from build123d import *

# Parameters (mm, degrees)
F1_DEPTH = 25.4
F3_DEPTH = 25.4
F4_W     = 29.7458320856
F4_H     = 10.7239410281
F4_W_2   = 77.620446682
F4_W_3   = 25.7802940905
F4_H_2   = 64.6573156118
F4_W_4   = 82.3989063501
F4_H_3   = 15.7408937812
F4_W_5   = 43.0548340082
F4_H_4   = 22.1842341125
F4_W_6   = 2.0285844803
F4_H_5   = 2.3600235581
F5_DEPTH = 25.4
F7_DEPTH = 25.4


with BuildPart() as f1:
    # F0 (on Front) → F1 (new body)
    with BuildSketch(Plane.XZ):
        Polygon((90.7035768032, 111.3269925117), (-373.5082440503, 867.1883240136), (-423.3669042587, 983.7029576302), (92.4958586693, -462.0907306671), (710.130751133, -1470.7733392715), (473.2221364975, -839.5437598228), align=None)
    extrude(amount=F1_DEPTH)

    # F2 (on face) → F3 (join)
    with BuildSketch(Plane(origin=(0, 0, 0), x_dir=(-1, 0, 0), z_dir=(0, 1, 0))):
        Polygon((-81.9063782692, 78.366830945), (-73.3345150948, 78.366830945), (-73.3345150948, 75.38125664), (0, 75.38125664), (0, 144.7913646698), (-146.6690301895, 144.7913646698), (-146.6690301895, 0), (-77.620446682, 0), (-77.620446682, 72.3956823349), (-81.9063782692, 72.3956823349), align=None)
        Polygon((0, 75.38125664), (-73.3345150948, 75.38125664), (-73.3345150948, 72.3956823349), (-77.620446682, 72.3956823349), (-77.620446682, 0), (0, 0), align=None)
        Polygon((77.620446682, 75.38125664), (0, 75.38125664), (0, 0), (-77.620446682, 0), (-77.620446682, -75.38125664), (77.620446682, -75.38125664), align=None)
    extrude(amount=F3_DEPTH)

    # F4 (on face) → F5 (join)
    with BuildSketch(Plane(origin=(0, 25.4, 0), x_dir=(-1, 0, 0), z_dir=(0, 1, 0))):
        with Locations((-14.8729160428, 70.0192861259)):
            Rectangle(F4_W, F4_H)
        Polygon((-43.309610337, 64.6573156118), (-29.7458320856, 64.6573156118), (-29.7458320856, 75.38125664), (-29.7458320856, 116.2622794509), (-112.1447384357, 116.2622794509), (-112.1447384357, 64.6573156118), (-69.0899044275, 64.6573156118), align=None)
        Polygon((0, 64.6573156118), (-29.7458320856, 64.6573156118), (-43.309610337, 64.6573156118), (-43.309610337, 0), (-43.309610337, -75.38125664), (77.620446682, -75.38125664), (77.620446682, 64.6573156118), align=None)
        with Locations((38.810223341, 70.0192861259)):
            Rectangle(F4_W_2, F4_H)
        Polygon((-29.7458320856, 116.2622794509), (-29.7458320856, 75.38125664), (0, 75.38125664), (0, 144.7913646698), (-29.7458320856, 144.7913646698), (-29.7458320856, 132.0031732321), align=None)
        with Locations((-56.1997573823, 32.3286578059)):
            Rectangle(F4_W_3, F4_H_2)
        with Locations((-70.9452852607, 124.1327263415)):
            Rectangle(F4_W_4, F4_H_3)
        with Locations((-90.6173214316, 32.3286578059)):
            Rectangle(F4_W_5, F4_H_2)
        Polygon((-112.1447384357, 64.6573156118), (-112.1447384357, 116.2622794509), (-128.1245350838, 116.2622794509), (-130.1531195641, 116.2622794509), (-130.1531195641, 64.6573156118), align=None)
        with Locations((-90.6173214316, -11.0921170563)):
            Rectangle(F4_W_5, F4_H_4)
        with Locations((-129.1388273239, 117.44229123)):
            Rectangle(F4_W_6, F4_H_5)
    extrude(amount=F5_DEPTH)

    # F6 (on face) → F7 (join)
    with BuildSketch(Plane(origin=(-77.620446682, 0, 0), x_dir=(0, -1, 0), z_dir=(-1, 0, 0))):
        Polygon((321.7040300369, 356.4623594284), (-374.66776371, 356.4623594284), (-204.5531272888, -290.0140881538), (321.7040300369, -362.3423576355), align=None)
    extrude(amount=F7_DEPTH)


solid = f1.part
Check sheet for the modelled part. Datum: model origin and axes. Units: mm. A direction names the side the tool comes from. Round coordinates to 2 decimals unless told otherwise and drop trailing zeros. Loops run counter-clockwise (first coordinate to the right, second up) from the corner with the lowest first, then second, coordinate; pieces in that order, holes last. Notation, with made-up numbers: M 16,-22.5 L 45,-22.5 A34 cw 45,10.5 Z; hole C 59,49 d4. An arc over 180 degrees is marked long. One line per question, with ' | ' between items. Start each with the question number.
Item 1: Section check A-A (z = -322). Record the boundary of the cut face in (x, y), and give its area (3 significant figures).
Item 2: Set-up check for faces 1 (the face through (28, 50.8, 36)), 2 (the face through (1, 25, -75.381)), 3 (the face through (-265.436, -12.522, 541.075)), 4 (the face through (-39, 25, 75.381)), 5 (the face through (126, 0, 89)): record each of +Z, -Z, +X, -X, +Y, -Y from which the full face is reachable in a straight line by a thin tool's end or side.
Item 3: Scan lines: probe 1 along X at (y, z) = (98, -171); probe 2 along Y at (x, z) = (-113.5, 147.5). Record each from-to range of solid material in increasing order.
Item 4: Release check for a two-part mould opening along X. For faces 6 (the face through (0, 25, 110)), 7 (the face through (396.99, -12.52, -959.37)), 8 (the face through (-90.14, -54.89, -325.67)), 9 (the face through (284.64, -12.52, -370.76)) record: released by +X, released by -X, zero draft, split by the parting line, or undercut.
Item 5: Section check C-C (y = 175.5). Record the boundary of the cut face in (x, z), and give its area (3 significant figures).
Item 6: Section check B-B (x = 513). Record the boundary of the cut face in (y, z), and give its area (3 significant figures).
Item 7: Gauge pin test, flat ends, axial feed: pin 1 Ø6 at (x, y) = (368, -13.5) entering from -Z; pin 2 Ø6.5 at (y, z) = (40.5, 138) entering from +X; pin 3 Ø2 at (y, z) = (-69, -325.5) entering from -X. Record the tip position at first contact, or that the pin passes through.
Worked out:
1) outline: M -103.02,-321.7 L -77.62,-321.7 L -77.62,-28.17 L -103.02,-28.17 Z; M 42.51,-25.4 L 265.02,-25.4 L 265.02,0 L 42.51,0 Z | area: 13,100 mm^2
2) face 1: +Z, -Z, +X, +Y | face 2: -Z, +X, +Y | face 3: -Z, -X, +Y, -Y | face 4: +Z, +Y | face 5: +Z, +X, -Y
3) probe 1: -103.02 to -77.62 | probe 2: -25.4 to 0
4) face 6: undercut | face 7: released by -X | face 8: zero draft | face 9: released by +X
5) outline: M -103.02,-294.01 L -77.62,-294.01 L -77.62,356.46 L -103.02,356.46 Z | area: 16,500 mm^2
6) outline: M -25.4,-1148.83 L 0,-1148.83 L 0,-945.53 L -25.4,-945.53 Z | area: 5,160 mm^2
7) pin 1: z = -916.93 | pin 2: x = 29.75 | pin 3: x = -103.02
